```python
from build123d import *

# Parameters (mm, degrees)
BOSS_EXTRU_1_DEPTH      = 7.5
BOSS_EXTRU_1_DEPTH_BACK = 15
ESQUISSE1_W             = 39
ESQUISSE1_H             = 30
BOSS_EXTRU_2_DEPTH      = 22.5
ESQUISSE3_W             = 24
ESQUISSE3_H             = 5
BOSS_EXTRU_3_DEPTH      = 10
ESQUISSE4_W             = 24
ESQUISSE4_H             = 5
BOSS_EXTRU_4_DEPTH      = 10
ESQUISSE5_W             = 24
ESQUISSE5_H             = 22.5
BOSS_EXTRU_5_DEPTH      = 10
ESQUISSE6_W             = 5
ESQUISSE6_H             = 10
ENL_V_MAT_EXTRU_1_DEPTH = 50.249365478
ESQUISSE7_W             = 8
ESQUISSE7_H             = 30
ENL_V_MAT_EXTRU_2_DEPTH = 15
ESQUISSE8_R             = 4
BOSS_EXTRU_6_DEPTH      = 25
ESQUISSE9_W             = 20
ESQUISSE9_H             = 10
ENL_V_MAT_EXTRU_3_DEPTH = 5


with BuildPart() as part:
    # Esquisse1 → Boss.-Extru.1 (new, two sides: drawn at the far end of the back side and taken through both)
    with BuildSketch(Plane(origin=(0, 0, 0), x_dir=(1, 0, 0), z_dir=(0, 1, 0)).offset(-BOSS_EXTRU_1_DEPTH_BACK)):
        Rectangle(ESQUISSE1_W, ESQUISSE1_H)
    extrude(amount=BOSS_EXTRU_1_DEPTH + BOSS_EXTRU_1_DEPTH_BACK)

    # Esquisse2 → Boss.-Extru.2 (add)
    with BuildSketch(Plane(origin=(0, 0, 0), x_dir=(1, 0, 0), z_dir=(0, 1, 0))):
        Polygon((-19.5, 0), (-19.5, 12), (-24.5, 12), (-24.5, -12), (-19.5, -12), align=None)
        Polygon((19.5, 0), (19.5, 12), (24.5, 12), (24.5, -12), (19.5, -12), align=None)
    extrude(amount=BOSS_EXTRU_2_DEPTH)

    # Esquisse3 → Boss.-Extru.3 (add)
    with BuildSketch(Plane(origin=(-19.5, 0, 0), x_dir=(0, 0, -1), z_dir=(1, 0, 0))):
        with Locations((0, 20)):
            Rectangle(ESQUISSE3_W, ESQUISSE3_H)
    extrude(amount=BOSS_EXTRU_3_DEPTH)

    # Esquisse4 → Boss.-Extru.4 (add)
    with BuildSketch(Plane.ZY.offset(-19.5)):
        with Locations((0, 20)):
            Rectangle(ESQUISSE4_W, ESQUISSE4_H)
    extrude(amount=BOSS_EXTRU_4_DEPTH)

    # Esquisse5 → Boss.-Extru.5 (add)
    with BuildSketch(Plane(origin=(24.5, 0, 0), x_dir=(0, 0, -1), z_dir=(1, 0, 0))):
        with Locations((0, 11.25)):
            Rectangle(ESQUISSE5_W, ESQUISSE5_H)
    extrude(amount=BOSS_EXTRU_5_DEPTH)

    # Esquisse6 → Enlèv. mat.-Extru.1 (cut, through all)
    with BuildSketch(Plane(origin=(0, 0, -12), x_dir=(-1, 0, 0), z_dir=(0, 0, -1))):
        with Locations((-27, 10)):
            Rectangle(ESQUISSE6_W, ESQUISSE6_H)
    extrude(amount=-ENL_V_MAT_EXTRU_1_DEPTH, mode=Mode.SUBTRACT)

    # Esquisse7 → Enlèv. mat.-Extru.2 (cut)
    with BuildSketch(Plane(origin=(0, 7.5, 0), x_dir=(1, 0, 0), z_dir=(0, 1, 0))):
        with Locations((-8, 0)):
            Rectangle(ESQUISSE7_W, ESQUISSE7_H)
        with Locations((8, 0)):
            Rectangle(ESQUISSE7_W, ESQUISSE7_H)
    extrude(amount=-ENL_V_MAT_EXTRU_2_DEPTH, mode=Mode.SUBTRACT)

    # Esquisse8 → Boss.-Extru.6 (add)
    with BuildSketch(Plane(origin=(-12, 0, 0), x_dir=(0, 0, -1), z_dir=(1, 0, 0))):
        with Locations(Location((0, 2.490962546, 0), (0, 0, 180))):
            Circle(ESQUISSE8_R)
    extrude(amount=BOSS_EXTRU_6_DEPTH)

    # Esquisse9 → Enlèv. mat.-Extru.3 (cut)
    with BuildSketch(Plane.XZ.offset(15)):
        Rectangle(ESQUISSE9_W, ESQUISSE9_H)
    extrude(amount=-ENL_V_MAT_EXTRU_3_DEPTH, mode=Mode.SUBTRACT)


solid = part.part
```
CAD build for the part. Positions are in the model's coordinates, mm. A direction names the side the tool comes from. Round coordinates to 2 decimals unless told otherwise and drop trailing zeros. Order: outer loops, then holes, each group sorted by start corner. A loop starts at its lowest first (then second) coordinate and runs counter-clockwise, first axis right, second up.
Q1. Slice it at A-A (y = -4). Write the cut outline in (x, z), and give its area (3 significant figures).
Q2. Slice it at B-B (x = -16). Write the cut outline in (y, z).
Q3. Drop flat-ended pins along their axis: pin 1 (7.5 mm diameter, centred on x = -18.5, y = 12, fed in from +Z); pin 2 (4 mm diameter, centred on x = 25, y = 9.5, fed in from -Z); pin 3 (3 mm diameter, centred on x = -4, z = 2, fed in from -Y). Give the stop position or say it passes through.
Q4. Slice it at C-C (z = 6.5). Write the cut outline in (x, y), and give its area (3 significant figures).
Q5. Which spindle directions (+Z, -Z, +X, -X, +Y, -Y) get a long thin tool onto all of the face, cutting with end or side? Do faces 4 (the flat face through (-9.5, 20, 0)), 5 (the flat face through (-20, 14, 12)), 6 (the flat face through (16, 7.5, 0)), 7 (the flat face through (0, -10, 0)), 8 (the flat face through (-12, -2, 0)). Say none if no direction does.
Q6. Slice it at D-D (y = 9.5). Write the cut outline in (x, z).
Q7. Wall check: L1, parallel to X at y = -0.5, z = -7; L2, parallel to X at y = 1.5, z = -9; L3, parallel to Y at x = 14, z = 7.25. Give the ranges that are in metal, low to high.
Q8. Two-plate mould, pull along Z, no slides. Class faces 1 (the flat face through (-19.5, -6, 0)), 2 (the flat face through (0, -13, 5)), 3 (the cylindrical face through (7.944, 4.925, -3.174)): pulls with the +Z half, pulls with the -Z half, needs draft (parallel to the pull), parting line crosses it, or undercut.
Results below:
1. outline: (-19.5, -15) - (-12, -15) - (-12, 15) - (-19.5, 15) - close; (-4, -15) - (4, -15) - (4, 15) - (-4, 15) - close; (12, -15) - (19.5, -15) - (19.5, 15) - (12, 15) - close
1. area: 690 mm2
2. outline: (-15, -15) - (7.5, -15) - (7.5, 15) - (-15, 15) - close; (17.5, -12) - (22.5, -12) - (22.5, 12) - (17.5, 12) - close
3. pin 1: stops at z = 12
3. pin 2: stops at z = -12
3. pin 3: stops at y = -10
4. outline: (-24.5, 0) - (-19.5, 0) - (-19.5, -15) - (19.5, -15) - (19.5, 0) - (34.5, 0) - (34.5, 22.5) - (9.5, 22.5) - (9.5, 17.5) - (19.5, 17.5) - (19.5, 7.5) - (12, 7.5) - (12, -7.5) - (4, -7.5) - (4, 7.5) - (-4, 7.5) - (-4, -7.5) - (-12, -7.5) - (-12, 7.5) - (-19.5, 7.5) - (-19.5, 17.5) - (-9.5, 17.5) - (-9.5, 22.5) - (-24.5, 22.5) - close; hole (24.5, 5) - (29.5, 5) - (29.5, 15) - (24.5, 15) - close
4. area: 1,140 mm2
5. face 4: +Z, -Z, +Y
5. face 5: +Z, -X, +Y
5. face 6: +Z, -Z
5. face 7: -Y
5. face 8: none
6. outline: (-24.5, -12) - (-19.5, -12) - (-19.5, 12) - (-24.5, 12) - close; (19.5, -12) - (24.5, -12) - (24.5, 12) - (19.5, 12) - close; (29.5, -12) - (34.5, -12) - (34.5, 12) - (29.5, 12) - close
7. L1: x = -19.5 to -12, -4 to 4, 12 to 19.5
7. L2: x = -24.5 to -12, -4 to 4, 12 to 34.5
7. L3: y = -15 to 7.5, 17.5 to 22.5
8. face 1: needs draft
8. face 2: undercut
8. face 3: parting line crosses it
